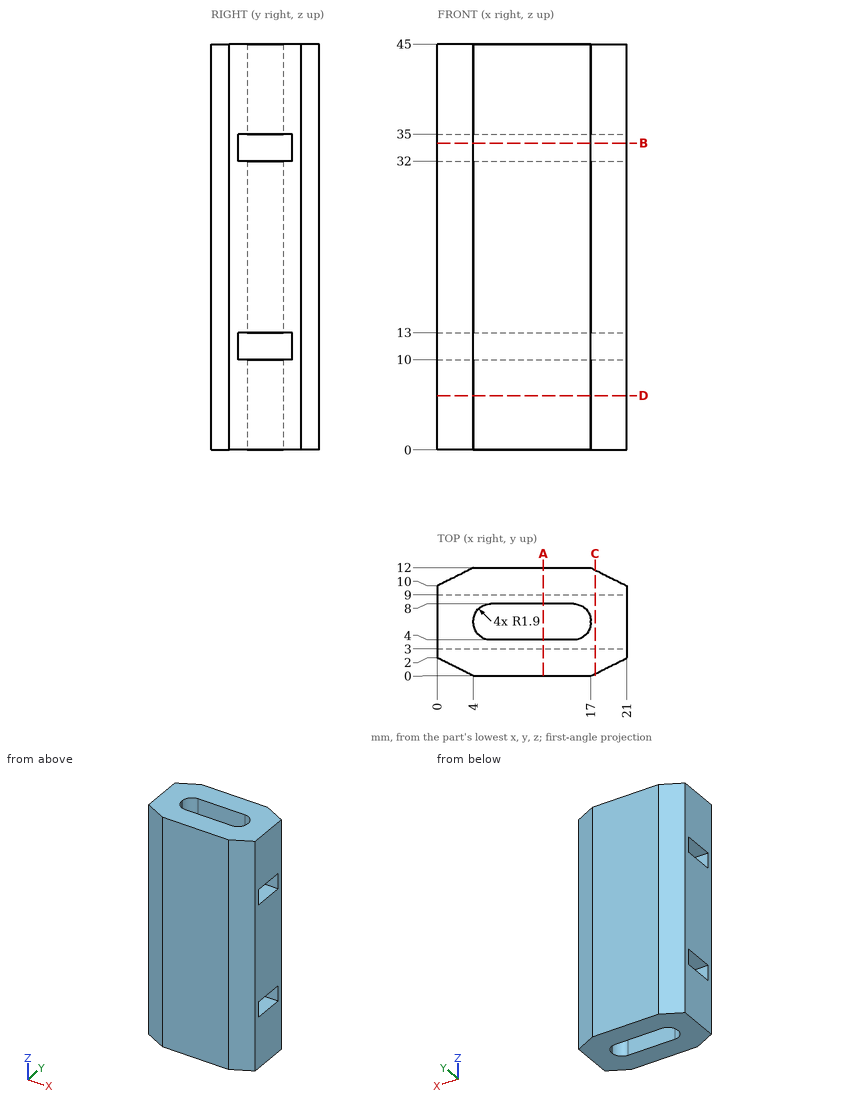
Geometry check sheet. Reference: drawing and pictorial views, mm from the part's lowest x, y, z. Give positions to 0.01 mm unless a question says otherwise; leave off trailing zeros. Order: outer loops, then holes, each group sorted by start corner. A loop starts at its lowest first (then second) coordinate and runs counter-clockwise, first axis right, second up. Notation, with made-up numbers: (23, 43.25) - (54, 43.25) arc R17 ccw to (54, 49.25) - close; hole circle Ø10 at (-7.5, 49). An arc over 180 degrees is marked (long way). Use one line per item in the form item = value.
1) Sectioned sample at D-D (z = 6). Record the boundary of the cut face in (x, y).
Working result:
outline = (0, 2) - (4, 0) - (17, 0) - (21, 2) - (21, 10) - (17, 12) - (4, 12) - (0, 10) - close; hole (4, 5.9) arc R1.9 ccw to (5.9, 4) - (15.1, 4) arc R1.9 ccw to (17, 5.9) - (17, 6.1) arc R1.9 ccw to (15.1, 8) - (5.9, 8) arc R1.9 ccw to (4, 6.1) - close
2) Depth check by flat-ended pin: pin 1 Ø1 at (x, y) = (7.5, 9) entering from -Z. Enter the tip coordinate at first touch or a pass-through.
Working result:
pin_1 = 0
3) Sectioned sample at B-B (z = 34). Record the boundary of the cut face in (x, y).
Working result:
outline = (0, 2) - (4, 0) - (17, 0) - (21, 2) - (21, 3) - (0, 3) - close; (0, 9) - (21, 9) - (21, 10) - (17, 12) - (4, 12) - (0, 10) - close
4) Sectioned sample at C-C (x = 17.5). Record the boundary of the cut face in (y, z).
Working result:
outline = (0.25, 0) - (11.75, 0) - (11.75, 45) - (0.25, 45) - close; hole (3, 10) - (9, 10) - (9, 13) - (3, 13) - close; hole (3, 32) - (9, 32) - (9, 35) - (3, 35) - close
5) Sectioned sample at A-A (x = 11.75). Record the boundary of the cut face in (y, z).
Working result:
outline = (0, 0) - (4, 0) - (4, 10) - (3, 10) - (3, 13) - (4, 13) - (4, 32) - (3, 32) - (3, 35) - (4, 35) - (4, 45) - (0, 45) - close; (8, 0) - (12, 0) - (12, 45) - (8, 45) - (8, 35) - (9, 35) - (9, 32) - (8, 32) - (8, 13) - (9, 13) - (9, 10) - (8, 10) - close
6) Material ranges on probe 1 along Z at (x, y) = (18.25, 7.75); probe 2 along Y at (x, z) = (8.25, 40); probe 3 along Y at (x, z) = (9.25, 34.5), recorded low to high. Write a range as from..to.
Working result:
probe_1 = 0..10, 13..32, 35..45
probe_2 = 0..4, 8..12
probe_3 = 0..3, 9..12
